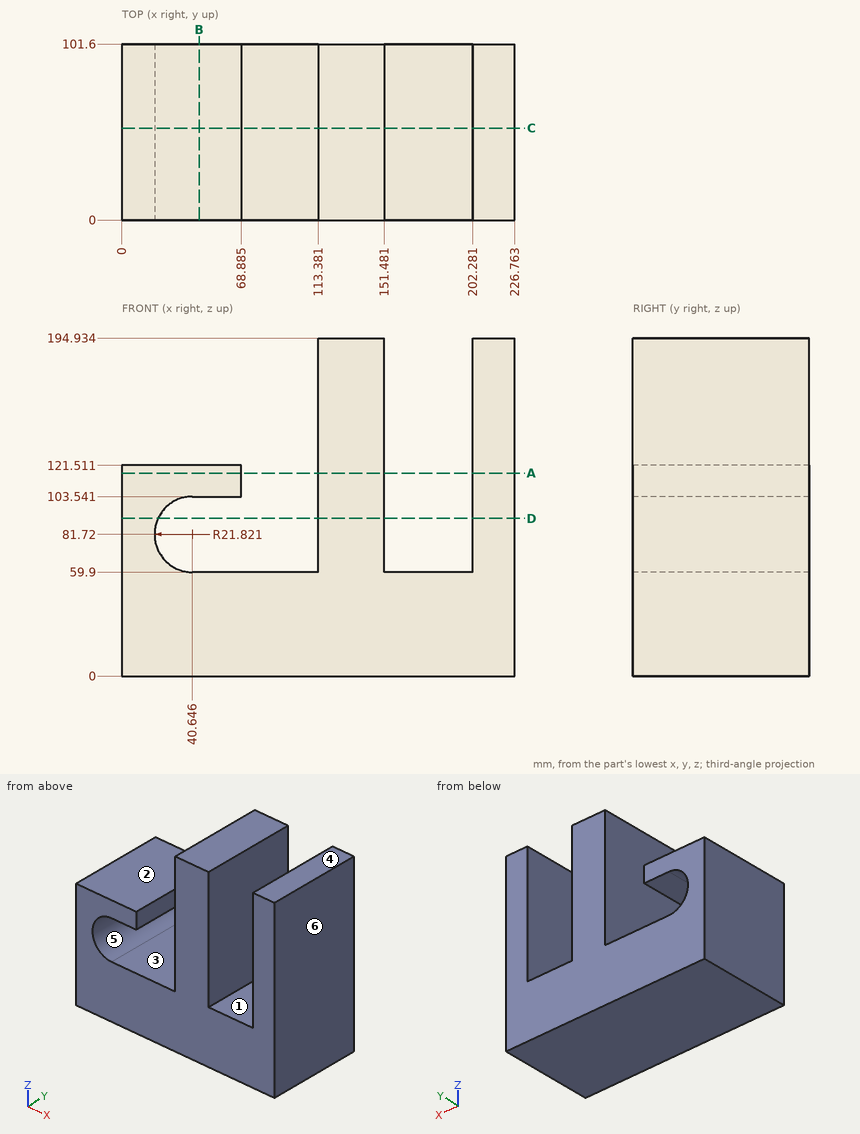
Design review of the part shown in the three views and the two pictorial views. Dimensions are in mm from the part's minimum x, y and z. A direction names the side the tool comes from. Round coordinates to 2 decimals unless told otherwise and drop trailing zeros. Order: outer loops, then holes, each group sorted by start corner. A loop starts at its lowest first (then second) coordinate and runs counter-clockwise, first axis right, second up.
Q1. Machinability: for the marked faces 1, 2 and 3, which of the approach directions +Z, -Z, +X, -X, +Y, -Y give a long, thin tool a straight path to every point of the face, cutting with its end or side? Answer none if there is none.
Findings below:
face 1: +Z, +Y, -Y
face 2: +Z, -X, +Y, -Y
face 3: +Y, -Y
Q2. Wall thickness on line 1 (X direction, y = 25.5, z = 115.5) (1 decimal); line 2 (X direction, y = 34, z = 91); line 3 (X direction, y = 69.5, z = 138): over which ranges is each line inside the solid? List them lowest first.
Findings below:
line 1: x = 0 to 68.9, 113.4 to 151.5, 202.3 to 226.8
line 2: x = 0 to 20.9, 113.38 to 151.48, 202.28 to 226.76
line 3: x = 113.38 to 151.48, 202.28 to 226.76
Q3. We need section B-B, the plane x = 44.5. Give the boundary of the cut face in (y, z).
Findings below:
outline: (0, 0) - (101.6, 0) - (101.6, 59.9) - (0, 59.9) - close; (0, 103.54) - (101.6, 103.54) - (101.6, 121.51) - (0, 121.51) - close
Q4. We need section A-A, the plane z = 117. Give the boundary of the cut face in (x, y) (1 decimal).
Findings below:
outline: (0, 0) - (68.9, 0) - (68.9, 101.6) - (0, 101.6) - close; (113.4, 0) - (151.5, 0) - (151.5, 101.6) - (113.4, 101.6) - close; (202.3, 0) - (226.8, 0) - (226.8, 101.6) - (202.3, 101.6) - close
Q5. Mouldability with a two-part tool opening along X and no side actions: class the marked faces 4, 5 and 6 as pulls with the +X half, pulls with the -X half, needs draft (parallel to the pull), parting line crosses it, or undercut.
Findings below:
face 4: needs draft
face 5: undercut
face 6: pulls with the +X half
Q6. Insertion check: P1, Ø2, axis at y = 40.5, z = 155, coming from the -X side; P2, Ø1, axis at x = 89, y = 50.5, coming from the +Z side. Each pin has a flat end and moves straight along its axis. Give the tip position at first contact, or say it passes through.
Findings below:
P1: stops at x = 113.38
P2: stops at z = 59.9
Q7. We need section C-C, the plane y = 53. Give the boundary of the cut face in (x, z) (1 decimal), plus the area to 3 significant figures.
Findings below:
outline: (0, 0) - (226.8, 0) - (226.8, 194.9) - (202.3, 194.9) - (202.3, 59.9) - (151.5, 59.9) - (151.5, 194.9) - (113.4, 194.9) - (113.4, 59.9) - (40.6, 59.9) arc R21.8 cw to (40.6, 103.5) - (68.9, 103.5) - (68.9, 121.5) - (0, 121.5) - close
area: 24,300 mm2
Q8. We need section D-D, the plane z = 91. Give the boundary of the cut face in (x, y).
Findings below:
outline: (0, 0) - (20.9, 0) - (20.9, 101.6) - (0, 101.6) - close; (113.38, 0) - (151.48, 0) - (151.48, 101.6) - (113.38, 101.6) - close; (202.28, 0) - (226.76, 0) - (226.76, 101.6) - (202.28, 101.6) - close
